For this review, use the dimensioned drawing (mm, ordinates from the lowest corner) and the shaded views. A direction names the side the tool comes from. Coordinates: 2 decimals unless noted, no trailing zeros. Loops run counter-clockwise (first coordinate to the right, second up) from the corner with the lowest first, then second, coordinate; pieces in that order, holes last. Notation, with made-up numbers: M -21,-34.5 L -7,-34.5 A20 ccw -7,-24.5 Z; hole C 12,73.25 d2. An arc over 180 degrees is marked long. One line per item, written item: value.
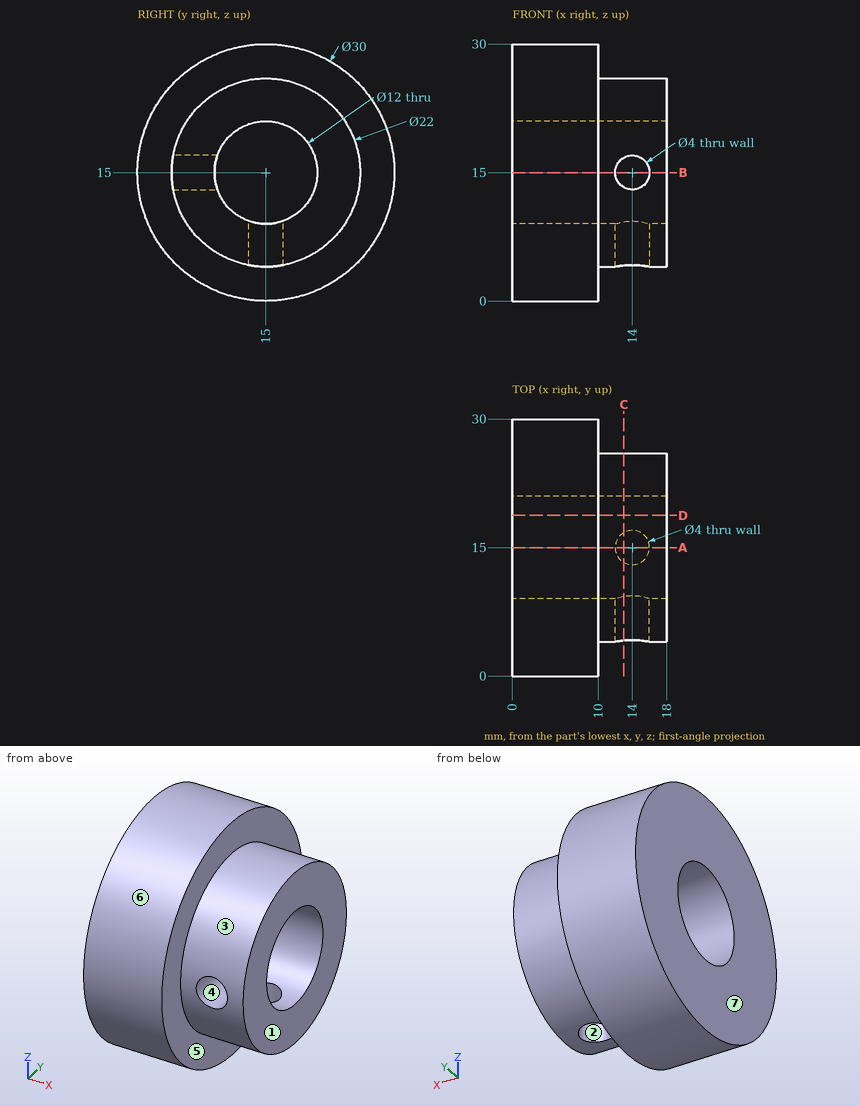
(1) Mouldability with a two-part tool opening along X and no side actions: class the marked faces 4, 5, 6 and 7 as released by +X, released by -X, zero draft, split by the parting line, or undercut.
Reply:
face 4: undercut
face 5: released by +X
face 6: zero draft
face 7: released by -X
(2) Insertion check: pin 1 (3.5 mm diameter, centred on x = 14, y = 15, fed in from +Z); pin 2 (3 mm diameter, centred on x = 13, y = 13.5, fed in from -Z); pin 3 (2 mm diameter, centred on x = 2.5, y = 9, fed in from +Z); pin 4 (10 mm diameter, centred on x = 11, y = 11.5, fed in from -Z). Each pin has a flat end and moves straight along its axis. Give the tip position at first contact, or say it passes through.
Reply:
pin 1: stops at z = 26
pin 2: stops at z = 4.01
pin 3: stops at z = 29.14
pin 4: stops at z = 0
(3) To check wall thickness, follow line 1 along Y through (x, z) = (8.75, 15); line 2 along X through (y, z) = (21.5, 2.75); line 3 along Y through (x, z) = (16.75, 12.5). State the ranges of each line that lie inside material, in increasing order. Write a range as [from, to].
Reply:
line 1: y = [0, 9], [21, 30]
line 2: x = [0, 10]
line 3: y = [4.29, 9.55], [20.45, 25.71]
(4) Tool access review of the marked faces 1, 2 and 3: name each direction out of +Z, -Z, +X, -X, +Y, -Y from which nothing blocks a thin tool from reaching the whole face with its end or side.
Reply:
face 1: +Z, -Z, +X, +Y, -Y
face 2: -Z
face 3: +X
(5) We need section A-A on y = 15. State the section outline as (x, z) points, then the cut area to 3 significant figures.
Reply:
outline: M 0,0 L 10,0 L 10,4 L 12,4 L 12,9 L 0,9 Z; M 0,21 L 18,21 L 18,26 L 10,26 L 10,30 L 0,30 Z; M 16,4 L 18,4 L 18,9 L 16,9 Z
area: 240 mm2
(6) We need section C-C on x = 13. State the section outline as (y, z) points.
Reply:
outline: M 4.14,13.27 A11 ccw 13.27,4.14 L 13.27,9.26 A6 cw 9.26,13.27 Z; M 4.14,16.73 L 9.26,16.73 A6 cw long 16.73,9.26 L 16.73,4.14 A11 ccw long Z
(7) We need section D-D on y = 18.75. State the section outline as (x, z) points, then the cut area to 3 significant figures.
Reply:
outline: M 0,0.48 L 10,0.48 L 10,4.66 L 18,4.66 L 18,10.32 L 0,10.32 Z; M 0,19.68 L 18,19.68 L 18,25.34 L 10,25.34 L 10,29.52 L 0,29.52 Z
area: 287 mm2
